Design review of the part built by this model. Coordinates are the model's own, in mm. A direction names the side the tool comes from. Give positions to 0.01 mm unless a question says otherwise; leave off trailing zeros. Order: outer loops, then holes, each group sorted by start corner. A loop starts at its lowest first (then second) coordinate and runs counter-clockwise, first axis right, second up.
```python
from build123d import *

# Parameters (mm, degrees)
BOSS_EXTRUDE1_DEPTH     = 38.1
SKETCH2_R               = 6.35
CUT_EXTRUDE1_DEPTH      = 277.034883433
ADVANCEDHOLE3_OUTLINE_R = 9.525
ADVANCEDHOLE3_DEPTH     = 38.1
SKETCH21_R              = 6.35
CUT_EXTRUDE2_DEPTH      = 35.56


# Read off the part's stored shape, not the designer's step: AdvancedHole3
with BuildPart() as part:
    # Sketch1 → Boss-Extrude1 (new body)
    with BuildSketch(Plane.XY):
        with BuildLine():
            Line((0, 0), (0, 203.013094366))
            ThreePointArc((0, 203.013094366), (50.8, 253.813094366), (101.6, 203.013094366))
            Line((101.6, 203.013094366), (101.6, 0))
            ThreePointArc((101.6, 0), (50.8, -50.8), (0, 0))
        make_face()
    extrude(amount=BOSS_EXTRUDE1_DEPTH)

    # Sketch2 → Cut-Extrude1 (cut, through all)
    with BuildSketch(Plane(origin=(101.6, 0, 0), x_dir=(0, 0, -1), z_dir=(1, 0, 0))):
        with Locations(Location((-19.05, 101.506547183, 0), (0, 0, 90))):
            Circle(SKETCH2_R)
    extrude(amount=-CUT_EXTRUDE1_DEPTH, mode=Mode.SUBTRACT)

    # AdvancedHole3 outline → AdvancedHole3 (cut)
    with BuildSketch(Plane.XY):
        with Locations((50.8, 203.013094366)):
            Circle(ADVANCEDHOLE3_OUTLINE_R)
        with Locations((50.8, 0)):
            Circle(ADVANCEDHOLE3_OUTLINE_R)
    extrude(amount=ADVANCEDHOLE3_DEPTH, mode=Mode.SUBTRACT)

    # Sketch21 → Cut-Extrude2 (cut)
    with BuildSketch(Plane.XY.offset(38.1)):
        with Locations((50.8, 50.706547183)):
            Circle(SKETCH21_R)
        with Locations((50.8, 152.213094366)):
            Circle(SKETCH21_R)
    extrude(amount=-CUT_EXTRUDE2_DEPTH, mode=Mode.SUBTRACT)


solid = part.part
```
1. Take a section at D-D (y = 54). State the section outline as (x, z) points.
Recorded:
outline: (0, 0) - (101.6, 0) - (101.6, 38.1) - (56.23, 38.1) - (56.23, 2.54) - (45.37, 2.54) - (45.37, 38.1) - (0, 38.1) - close
2. Take a section at B-B (z = 19.05). State the section outline as (x, y) points (3 decimals), then the cut area to 3 significant figures.
Recorded:
outline: (0, 0) arc R50.8 ccw to (101.6, 0) - (101.6, 95.157) - (0, 95.157) - close; (0, 107.857) - (101.6, 107.857) - (101.6, 203.013) arc R50.8 ccw to (0, 203.013) - close; hole circle Ø19.05 at (50.8, 0); hole circle Ø19.05 at (50.8, 203.013); hole circle Ø12.7 at (50.8, 50.707); hole circle Ø12.7 at (50.8, 152.213)
area: 26,600 mm2
3. Take a section at A-A (x = 50.8). State the section outline as (y, z) points (3 decimals), then the cut area to 3 significant figures.
Recorded:
outline: (-50.8, 0) - (-9.525, 0) - (-9.525, 38.1) - (-50.8, 38.1) - close; (9.525, 0) - (193.488, 0) - (193.488, 38.1) - (158.563, 38.1) - (158.563, 2.54) - (145.863, 2.54) - (145.863, 38.1) - (57.057, 38.1) - (57.057, 2.54) - (44.357, 2.54) - (44.357, 38.1) - (9.525, 38.1) - close; (212.538, 0) - (253.813, 0) - (253.813, 38.1) - (212.538, 38.1) - close; hole circle Ø12.7 at (101.507, 19.05)
area: 9,120 mm2
4. Draft analysis for pull direction Y (two halves, no side actions). For faces 3 (the face through (101.6, 103, 27)), 4 (the face through (51, 51, 2.54)), 5 (the face through (49.7, 253.8, 18.8)), state which applies: pulls with the +Y half, pulls with the -Y half, needs draft (parallel to the pull), parting line crosses it, or undercut.
Recorded:
face 3: needs draft
face 4: undercut
face 5: pulls with the +Y half
5. Take a section at C-C (x = 85). State the section outline as (y, z) points, then the cut area to 3 significant figures.
Recorded:
outline: (-37.56, 0) - (240.58, 0) - (240.58, 38.1) - (-37.56, 38.1) - close; hole circle Ø12.7 at (101.51, 19.05)
area: 10,500 mm2
6. For pin 1 (5 mm diameter, centred on x = 20.5, z = 14, fed in from +Y); pin 2 (10 mm diameter, centred on x = 88.5, z = 5.5, fed in from -Y), all flat-tipped, find the tip position at first contact; note any pin that passes through.
Recorded:
pin 1: stops at y = 245.53
pin 2: stops at y = -38.88
7. For line 1 along Y through (x, z) = (50.8, 10.5) (3 decimals); line 2 along X through (y, z) = (51.5, 16.5); line 3 along Y through (x, z) = (50, 16), list the stretches that pass through material, from the lowest coordinate up.
Recorded:
line 1: y = -50.8 to -9.525, 9.525 to 44.357, 57.057 to 145.863, 158.563 to 193.488, 212.538 to 253.813
line 2: x = 0 to 44.5, 57.1 to 101.6
line 3: y = -50.79 to -9.49, 9.49 to 44.41, 57.01 to 95.94, 107.08 to 145.91, 158.51 to 193.52, 212.5 to 253.81
8. Machinability: for faces 1 (the face through (59.6, -3.65, 18.78)), 2 (the face through (53.73, 45.073, 20.569)), which of the approach directions +Z, -Z, +X, -X, +Y, -Y give a long, thin tool a straight path to every point of the face, cutting with its end or side? Answer none if there is none.
Recorded:
face 1: +Z, -Z
face 2: +Z
